Input: part model. Units: mm. Frame: model coordinates. A direction names the side the tool comes from. Give positions to 0.01 mm unless a question says otherwise; leave off trailing zeros. Order: outer loops, then holes, each group sorted by start corner. A loop starts at its lowest first (then second) coordinate and runs counter-clockwise, first axis right, second up. Notation, with made-up numbers: M 31,73.5 L 44,73.5 A19 cw 44,81.5 Z; hole C 39,52 d5. An arc over 180 degrees is marked long. Use a Markdown table: item, result.
Autodesk Inventor part; units mm, degrees
ref_plane "YZ Plane" through (0, 0, 0) normal (1, 0, 0) x (0, 1, 0)
ref_plane "XZ Plane" through (0, 0, 0) normal (0, 1, 0) x (-1, 0, 0)
ref_plane "XY Plane" through (0, 0, 0) normal (0, 0, 1) x (1, 0, 0)
sketch "スケッチ1" plane through (0, 0, 0) normal (0, 0, 1) x (1, 0, 0)
  line L0 (-32.25, 31) -> (32.25, 31)
  line L1 (32.25, 31) -> (32.25, -31)
  line L2 (32.25, -31) -> (10, -31)
  line L3 (-32.25, -31) -> (-32.25, 31)
  line L4 (-32.25, 31) -> (32.25, -31) construction
  line L5 (32.25, 31) -> (-32.25, -31) construction
  line L6 (-29.25, 28.5) -> (29.25, 28.5)
  line L7 (29.25, 28.5) -> (29.25, -28.5)
  line L8 (29.25, -28.5) -> (12.5, -28.5)
  line L9 (-29.25, -28.5) -> (-29.25, 28.5)
  line L10 (-29.25, 28.5) -> (29.25, -28.5) construction
  line L11 (29.25, 28.5) -> (-29.25, -28.5) construction
  line L12 (0, 31) -> (0, -28.25) construction
  line L13 (-10, -31) -> (-10, -21)
  line L14 (-10, -21) -> (10, -21)
  line L15 (10, -31) -> (10, -21)
  line L16 (-12.5, -28.5) -> (-12.5, -18.5)
  line L17 (-12.5, -18.5) -> (12.5, -18.5)
  line L18 (12.5, -28.5) -> (12.5, -18.5)
  line L19 (-12.5, -28.5) -> (-29.25, -28.5)
  line L20 (-10, -31) -> (-32.25, -31)
  line L21 (-10, -31) -> (10, -31)
  point P0 (0, 0)
  point P1 (10, -25.75)
  point P2 (10, -28.25)
  point P3 (-10, -25.75)
  dimension "d0" = 64.5
  dimension "d1" = 62
  dimension "d2" = 3
  dimension "d3" = 2.5
  dimension "d40" = 20
  dimension "d41" = 10
  dimension "d42" = 2.5
  dimension "d43" = 2.5
extrude "押し出し1" add sketch "スケッチ1" along normal blind 5 contours L0 L1 L2 L15 L14 L13 L20 L3
extrude "押し出し2" add sketch "スケッチ1" along normal blind 1 contours L13 L14 L15 L21 | L6 L7 L8 L18 L17 L16 L19 L9
sketch "スケッチ2" plane through (32.25, -31, 0) normal (1, 0, 0) x (0, 0, -1)
  line L0 (0, 0) -> (-5, 0)
  line L1 (0, 62) -> (-5, 62)
  line L2 (-2.5, 62) -> (-2.5, 0) construction
  point P0 (0, 31)
  point P1 (-2.5, 59.5)
  point P2 (-2.5, 5)
  point P3 (-2.5, 10)
  dimension "d8" = 5
  dimension "d9" = 5
  dimension "d10" = 2.5
hole "穴1" at (32.25, 28.5, 2.5) direction (-1, 0, 0) diameter 3 depth 2.9
hole "穴2" at (32.25, -21, 2.5) at (32.25, -26, 2.5) direction (-1, 0, 0) diameter 2.8 depth 3
fillet "フィレット1" radius 2 12 edges at (-29.25, 28.5, 3) (29.25, -28.5, 3) (29.25, 28.5, 3) (-12.5, -28.5, 3) (-29.25, -28.5, 3) (12.5, -28.5, 3) (10, -21, 3) (-10, -21, 3) (-12.5, -18.5, 3) (12.5, -18.5, 3) (-10, -31, 3) (10, -31, 3)
sketch "スケッチ3" plane through (-32.25, -31, 0) normal (-1, 0, 0) x (0, 0, 1)
  circle A0 centre (2.5, 59.5) radius 1.5
  arc A1 (3.8077, 4.5) -> (1.1923, 4.5) centre (2.5, 5) ccw
  circle A2 centre (2.5, 10) radius 1.4
  point P0 (0, 31)
  point P1 (2.5, 5)
  point P2 (2.5, 10)
hole "穴3" at (-32.25, 28.5, 2.5) direction (1, 0, 0) diameter 3 depth 2.9
hole "穴4" at (-32.25, -26, 2.5) at (-32.25, -21, 2.5) direction (1, 0, 0) diameter 2.8 depth 3
equation "\"d43\" = d42"
properties part number "Cockpit_upper_back_door" material "アセタール樹脂、黒"
1) Cut plane C-C on z = 2.5. State how many separate pieces and enclosed holes the cut face has, and give its area (3 significant figures).
Response values:
| item | result |
|---|---|
| separate pieces | 4 |
| enclosed holes | 0 |
| area | 667 mm² |
2) Material intervals for line 1 (Y direction, x = -29.85, z = 2.5); line 2 (X direction, y = 3, z = 3.95); line 3 (Y direction, x = 17.5, z = 4.75), sorted ascending. Write a range as from..to.
Response values:
| item | result |
|---|---|
| line 1 | y = -31..-27.4, -24.6..-22.4, -19.6..27, 30..31 |
| line 2 | x = -32.25..-29.25, 29.25..32.25 |
| line 3 | y = -31..-28.5, 28.5..31 |
3) Mould query, pull axis Y, two halves, no side actions, for faces 1 (the face through (32.25, 0, 2)), 2 (the face through (9.4, -21.57, 2.97)), 3 (the face through (21, -28.5, 3)). Classes: released by +Y, released by -Y, zero draft, split by the parting line, or undercut.
Response values:
| item | result |
|---|---|
| face 1 | zero draft |
| face 2 | released by -Y |
| face 3 | undercut |
4) Cut plane A-A on y = -17. Return loops of the section in (x, z), and give its area (3 significant figures).
Response values:
| item | result |
|---|---|
| outline | M -32.25,0 L 32.25,0 L 32.25,5 L 29.25,5 L 29.25,1 L -29.25,1 L -29.25,5 L -32.25,5 Z |
| area | 88.5 mm² |
5) Reachability of faces 4 (the face through (-30.729, -19.633, 2.197)), 5 (the face through (-10.57, -30.4, 2.97)), 6 (the face through (29.25, 0, 3)) from +Z, -Z, +X, -X, +Y, -Y: full face, straight path, thin tool, end or side. Return the list, or none.
Response values:
| item | result |
|---|---|
| face 4 | -X |
| face 5 | +Z, -Y |
| face 6 | +Z |
6) Cut plane B-B on x = -16.5. Return loops of the section in (y, z), and give its area (3 significant figures).
Response values:
| item | result |
|---|---|
| outline | M -31,0 L 31,0 L 31,5 L 28.5,5 L 28.5,1 L -28.5,1 L -28.5,5 L -31,5 Z |
| area | 82.0 mm² |
7) First-contact query: pin 1 Ø11 at (x, y) = (-4, -27.5) entering from +Z; pin 2 Ø2 at (y, z) = (-26, 2.5) entering from +X. Flat tips, straight axial feed; report the tip coordinate or a pass-through.
Response values:
| item | result |
|---|---|
| pin 1 | stops at z = 1 |
| pin 2 | stops at x = 12.56 |
